```python
from build123d import *

# Parameters (mm, degrees)
SKETCH1_R               = 6.5
BOSS_EXTRUDE1_DEPTH     = 3
SKETCH4_R               = 4.5
CUT_EXTRUDE1_DEPTH      = 0.8
CUT_EXTRUDE2_DEPTH      = 10.669539803
CUT_EXTRUDE2_DEPTH_BACK = 10.669539803
SKETCH5_R               = 2.5


with BuildPart() as part:
    # Sketch1 → Boss-Extrude1 (new, symmetric)
    with BuildSketch(Plane(origin=(0, 0, 0), x_dir=(0, 0, -1), z_dir=(1, 0, 0))):
        Circle(SKETCH1_R)
    extrude(amount=BOSS_EXTRUDE1_DEPTH, both=True)

    # Sketch2 → Cut-Revolve1 (revolve, cut)
    with BuildSketch(Plane.XY, mode=Mode.PRIVATE) as cut_revolve1_sk:
        Polygon((-2, 6.5), (0, 4.5), (2, 6.5), align=None)
    revolve(cut_revolve1_sk.sketch.rotate(Axis((3, 0, 0), (-1, 0, 0)), 90), axis=Axis((3, 0, 0), (-1, 0, 0)), mode=Mode.SUBTRACT)

    # Sketch4 → Cut-Extrude1 (cut)
    with BuildSketch(Plane(origin=(3, 0, 0), x_dir=(0, 0, -1), z_dir=(1, 0, 0))):
        Circle(SKETCH4_R)
    cut_extrude1 = extrude(amount=-CUT_EXTRUDE1_DEPTH, mode=Mode.SUBTRACT)

    # Mirror1: Cut-Extrude1 across plane
    add(cut_extrude1.mirror(Plane(origin=(0, 0, 0), x_dir=(0, 0, 1), z_dir=(1, 0, 0))), mode=Mode.SUBTRACT)

    # Sketch5 → Cut-Extrude2 (cut, two sides: drawn at the far end of the back side and taken through both)
    with BuildSketch(Plane(origin=(0, 0, 0), x_dir=(0, 0, -1), z_dir=(1, 0, 0)).offset(-CUT_EXTRUDE2_DEPTH_BACK)):
        Circle(SKETCH5_R)
    extrude(amount=CUT_EXTRUDE2_DEPTH + CUT_EXTRUDE2_DEPTH_BACK, mode=Mode.SUBTRACT)


solid = part.part
```
Read the model definition and answer for the solid it produces. Units are mm, in the model's axes. A direction names the side the tool comes from. Give positions to 0.01 mm unless a question says otherwise; leave off trailing zeros. Order: outer loops, then holes, each group sorted by start corner. A loop starts at its lowest first (then second) coordinate and runs counter-clockwise, first axis right, second up. Notation, with made-up numbers: (3, 88.5) -> (43, 88.5) arc R28 ccw to (43, 124.5) -> close; hole circle Ø9 at (-33, -16.75). An arc over 180 degrees is marked (long way). Write item = value, one per line.
1. A cutting plane is placed at A-A, the plane z = 0. Write down the section's boundary in (x, y), and give its area (3 significant figures).
Numbers:
outline = (-3, -6.5) -> (-2, -6.5) -> (0, -4.5) -> (2, -6.5) -> (3, -6.5) -> (3, -4.5) -> (2.2, -4.5) -> (2.2, -2.5) -> (-2.2, -2.5) -> (-2.2, -4.5) -> (-3, -4.5) -> close; (-3, 4.5) -> (-2.2, 4.5) -> (-2.2, 2.5) -> (2.2, 2.5) -> (2.2, 4.5) -> (3, 4.5) -> (3, 6.5) -> (2, 6.5) -> (0, 4.5) -> (-2, 6.5) -> (-3, 6.5) -> close
area = 33.6 mm²
2. A cutting plane is placed at D-D, the plane x = -0.8. Write down the section's boundary in (y, z).
Numbers:
outline = circle Ø10.6 at (0, 0); hole circle Ø5 at (0, 0)
3. The mould has two halves that part along X. Classify faces 1 (the face through (0.13, 4.52, 1)), 2 (the face through (2.507, -3.955, 5.158)), 3 (the face through (-2.2, -2, -2)): +X half, -X half, draft (parallel to the pull), parting line (faces both ways), or undercut.
Numbers:
face_1 = undercut
face_2 = draft
face_3 = -X half
4. Given pin 1 (5.5 mm diameter, centred on y = 0, z = 0, fed in from -X); pin 2 (1.5 mm diameter, centred on x = 2.5, y = -3, fed in from -Z); pin 3 (2 mm diameter, centred on x = 2, z = 5, fed in from +Y); pin 4 (7 mm diameter, centred on y = 2, z = -2, fed in from +X), each flat-ended and moving along its own axis, determine where each tip first touches the part or whether it passes through.
Numbers:
pin_1 = -2.2
pin_2 = -6.1
pin_3 = 5.12
pin_4 = 3
5. For faces 4 (the face through (-2.61, 4.46, 0.59)), 5 (the face through (2.2, -2, -2)), 6 (the face through (-0.03, -2.44, 0.54)), determine the directions among +Z, -Z, +X, -X, +Y, -Y from which every point of the face is accessible in a straight line to the end or side of a thin tool.
Numbers:
face_4 = -X
face_5 = +X
face_6 = +X, -X
6. A cutting plane is placed at C-C, the plane x = 0.65. Write down the section's boundary in (y, z).
Numbers:
outline = circle Ø10.3 at (0, 0); hole circle Ø5 at (0, 0)
7. Straight lines are drawn through the part: line 1 along Y through (x, z) = (-2.35, 0); line 2 along Z through (x, y) = (1.8, -2.25); line 3 along X through (y, z) = (-1.5, -6). For each, find the intervals that lie inside material, in ascending order.
Numbers:
line_1 = -6.5 to -4.5, 4.5 to 6.5
line_2 = -5.88 to -1.09, 1.09 to 5.88
line_3 = -3 to -1.68, 1.68 to 3
